Part model, mm, in its own coordinate system. A direction names the side the tool comes from. Coordinates: 2 decimals unless noted, no trailing zeros. Loops run counter-clockwise (first coordinate to the right, second up) from the corner with the lowest first, then second, coordinate; pieces in that order, holes last. Notation, with made-up numbers: (4, 71) - (33, 71) arc R19 cw to (33, 104) - close; hole circle Ø3 at (-37.75, 72). An arc over 180 degrees is marked (long way). Use a Markdown table: item, result. Add a question column.
1. Band-saw the part on C-C, the plane y = -6. Give the cut face in (x, z), plus the area to 3 significant figures.
2. Wall check: probe 1 along Z at (x, y) = (60, -7.5); probe 2 along X at (y, z) = (0.25, 17); probe 3 along X at (y, z) = (0, 19). Give the ranges that are in metal, low to high. Write a range as [from, to].
3. 3-axis set-ups, long thin cutter, end or side, ignore diameter. For faces 4 (the flat face through (68.58, -8, 16)), 5 (the flat face through (-48, -2.54, 27)), 6 (the flat face through (50, 0, 22.296)), 7 (the flat face through (70, 0, 12.7)), 8 (the flat face through (-58, -8.3, 12.7)): which of +Z, -Z, +X, -X, +Y, -Y reach the whole face in a straight line?
4. Pull direction X, two halves, no side cores. Call faces 1 (the flat face through (-76.2, -4, 19)), 2 (the flat face through (67, -3, 17.78)), 3 (the flat face through (-1, -12.7, 15)): pulls with the +X half, pulls with the -X half, needs draft (parallel to the pull), parting line crosses it, or undercut.
5. Band-saw the part on A-A, the plane y = 0. Give the cut face in (x, z).
6. Band-saw the part on B-B, the plane x = 51. Give the cut face in (y, z).
7. Drop flat-ended pins along their axis: pin 1 (6.5 mm diameter, centred on y = -2, z = 5, fed in from -X); pin 2 (4 mm diameter, centred on y = 3, z = 28.5, fed in from -X). Give the stop position or say it passes through.
8. Band-saw the part on D-D, the plane z = 7. Give the cut face in (x, y), plus the area to 3 significant figures.
from build123d import *

# Parameters (mm, degrees)
F1_W      = 152.4
F1_H      = 25.4
F2_DEPTH  = 25.4
F3_R      = 9.8472712537
F4_DEPTH  = 25.401
F5_W      = 25.4
F5_H      = 12.7
F6_DEPTH  = 25.4
F7_W      = 25.4
F7_H      = 2.5977271069
F8_DEPTH  = 53.086
F9_W      = 128.2310737193
F9_H      = 25.4
F10_DEPTH = 5.08
F11_R     = 7.62
F12_W     = 5.08
F12_H     = 2.54
F13_DEPTH = 6.35508
F14_W     = 0.2449715817
F14_H     = 2.54
F15_DEPTH = 1.27
F14_W_2   = 0.2464826526
F16_DEPTH = 1.27
F17_W     = 5.08
F17_H     = 5.08
F18_DEPTH = 12.7
F19_W     = 5.08
F19_H     = 2.54
F20_DEPTH = 25.4


with BuildPart() as f2:
    # F1 (on face) → F2 (new body)
    with BuildSketch(Plane.XY):
        Rectangle(F1_W, F1_H)
    extrude(amount=F2_DEPTH)

    # F3 (on face) → F4 (cut, through all)
    with BuildSketch(Plane.XY):
        with Locations((-63.8753846288, 0)):
            Circle(F3_R)
    extrude(amount=F4_DEPTH, mode=Mode.SUBTRACT)

    # F5 (on face) → F6 (cut)
    with BuildSketch(Plane(origin=(-76.2, 0, 0), x_dir=(0, -1, 0), z_dir=(-1, 0, 0))):
        with Locations((0, 6.35)):
            Rectangle(F5_W, F5_H)
    extrude(amount=-F6_DEPTH, mode=Mode.SUBTRACT)

    # F7 (on face) → F8 (cut)
    with BuildSketch(Plane(origin=(0, 12.7, 0), x_dir=(-1, 0, 0), z_dir=(0, 1, 0))):
        with Locations((-49.7299730778, 20.9970995784)):
            Rectangle(F7_W, F7_H)
    extrude(amount=-F8_DEPTH, mode=Mode.SUBTRACT)

    # F9 (on face) → F10 (join)
    with BuildSketch(Plane.XY.offset(25.4)):
        with Locations((12.0844631404, 0)):
            Rectangle(F9_W, F9_H)
    extrude(amount=F10_DEPTH)

    # F11
    f11_edges = [f2.edges().sort_by_distance(p)[0] for p in [
        (-76.2, 12.7, 19.05),
    ]]
    fillet(f11_edges, radius=F11_R)

    # F12 (on face) → F13 (cut)
    with BuildSketch(Plane(origin=(-52.0310737193, 0, 0), x_dir=(0, -1, 0), z_dir=(-1, 0, 0))):
        with Locations((0, 26.67)):
            Rectangle(F12_W, F12_H)
    extrude(amount=-F13_DEPTH, mode=Mode.SUBTRACT)

    # F14 (on face) → F15 (join)
    with BuildSketch(Plane(origin=(-52.0310737193, 0, 0), x_dir=(0, -1, 0), z_dir=(-1, 0, 0))):
        with Locations((-2.4175142092, 26.67)):
            Rectangle(F14_W, F14_H)
    extrude(amount=-F15_DEPTH)

    # F14 (on face) → F16 (join)
    with BuildSketch(Plane(origin=(-52.0310737193, 0, 0), x_dir=(0, -1, 0), z_dir=(-1, 0, 0))):
        with Locations((2.4167586737, 26.67)):
            Rectangle(F14_W_2, F14_H)
    extrude(amount=-F16_DEPTH)

    # F17 (on face) → F18 (cut)
    with BuildSketch(Plane.YZ.offset(76.2)):
        with Locations((0, 15.24)):
            Rectangle(F17_W, F17_H)
    extrude(amount=-F18_DEPTH, mode=Mode.SUBTRACT)

    # F19 (on face) → F20 (cut)
    with BuildSketch(Plane(origin=(0, -2.54, 0), x_dir=(-1, 0, 0), z_dir=(0, 1, 0))):
        with Locations((-66.04, 16.51)):
            Rectangle(F19_W, F19_H)
    extrude(amount=-F20_DEPTH, mode=Mode.SUBTRACT)


solid = f2.part
Geometry check:
| question | item | result |
|---|---|---|
| 1 | outline | (-76.2, 12.7) - (-71.68, 12.7) - (-71.68, 25.4) - (-76.2, 25.4) - close; (-56.07, 12.7) - (-50.8, 12.7) - (-50.8, 0) - (76.2, 0) - (76.2, 30.48) - (-52.03, 30.48) - (-52.03, 25.4) - (-56.07, 25.4) - close; hole (37.03, 19.7) - (62.43, 19.7) - (62.43, 22.3) - (37.03, 22.3) - close; hole (63.5, 15.24) - (68.58, 15.24) - (68.58, 17.78) - (63.5, 17.78) - close |
| 1 | area | 3,920 mm^2 |
| 2 | probe 1 | z = [0, 19.7], [22.3, 30.48] |
| 2 | probe 2 | x = [-76.2, -73.72], [-54.03, 63.5] |
| 2 | probe 3 | x = [-76.2, -73.72], [-54.03, 76.2] |
| 3 | face 4 | -Y |
| 3 | face 5 | none |
| 3 | face 6 | +Y, -Y |
| 3 | face 7 | +X |
| 3 | face 8 | -Z, -X, +Y, -Y |
| 4 | face 1 | pulls with the -X half |
| 4 | face 2 | undercut |
| 4 | face 3 | needs draft |
| 5 | outline | (-76.2, 12.7) - (-73.72, 12.7) - (-73.72, 25.4) - (-76.2, 25.4) - close; (-54.03, 12.7) - (-50.8, 12.7) - (-50.8, 0) - (76.2, 0) - (76.2, 12.7) - (63.5, 12.7) - (63.5, 17.78) - (76.2, 17.78) - (76.2, 30.48) - (-52.03, 30.48) - (-52.03, 27.94) - (-45.68, 27.94) - (-45.68, 25.4) - (-54.03, 25.4) - close; hole (37.03, 19.7) - (62.43, 19.7) - (62.43, 22.3) - (37.03, 22.3) - close |
| 6 | outline | (-12.7, 0) - (12.7, 0) - (12.7, 19.7) - (-12.7, 19.7) - close; (-12.7, 22.3) - (12.7, 22.3) - (12.7, 30.48) - (-12.7, 30.48) - close |
| 7 | pin 1 | stops at x = -50.8 |
| 7 | pin 2 | stops at x = -52.03 |
| 8 | outline | (-50.8, -12.7) - (76.2, -12.7) - (76.2, 12.7) - (-50.8, 12.7) - close |
| 8 | area | 3,230 mm^2 |
